Can you work these out from the model? Positions are in its coordinate system, mm. Face numbers are marked on the shaded views. Round coordinates to 2 decimals unless told otherwise and drop trailing zeros. Order: outer loops, then holes, each group sorted by start corner. A loop starts at its lowest first (then second) coordinate and runs counter-clockwise, first axis right, second up. Notation, with made-up numbers: (38.25, 8) -> (53.25, 8) arc R18 ccw to (53.25, 29) -> close; hole circle Ø8 at (11, -3). An arc over 180 degrees is marked (long way). Use a Markdown table: item, result. Add a question column.
Q1. If we section it at B-B on z = -4: List the corners of the cut face in (x, y) for me.
Q2. I need wall thicknesses on line 1 along Y through (x, z) = (0, -7.5); line 2 along Z through (x, y) = (0.05, 0.5); line 3 along Z through (x, y) = (-0.7, -1.6). Which ranges of each line are inside material? Lowest first, please. Write a range as [from, to].
Q3. We'd pull the mould along X, two halves only. Please class the marked faces 1, 2, 3 and 4: +X half, -X half, draft (parallel to the pull), parting line (faces both ways), or undercut.
Q4. If we section it at D-D on z = 7.75: List the corners of the cut face in (x, y) for me.
Q5. If we section it at C-C on y = 0.6: List the corners of the cut face in (x, z) for me.
Q6. If we section it at A-A on x = 0: List the corners of the cut face in (y, z) for me.
Q7. I'm going to push flat-ended pins straight in: pin 1 Ø1.5 at (x, y) = (2, 1.5) entering from +Z; pin 2 Ø0.8 at (x, y) = (0, -0.5) entering from -Z; pin 3 Ø2 at (y, z) = (0.5, -10) entering from +X. Where does each tip first touch, or does it pass through?
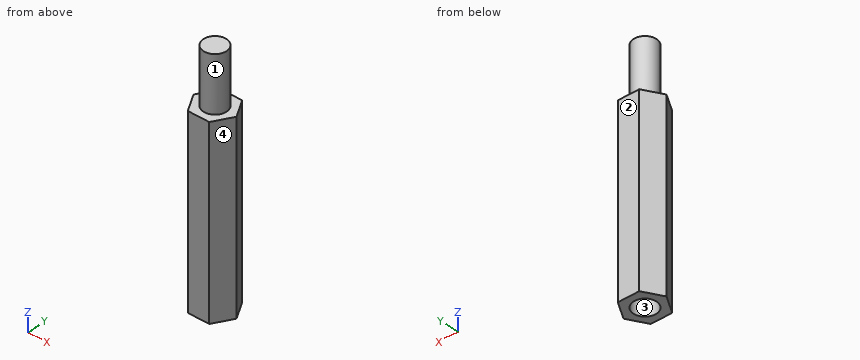
Autodesk Fusion 360 part; units mm, degrees
sketch "Sketch1" plane through (0, 0, 0) normal (0, 0, 1) x (1, 0, 0)
  circle A0 centre (0, 0) radius 1.25
  line L0 (2.3094, 0) -> (1.1547, 2)
  line L1 (1.1547, 2) -> (-1.1547, 2)
  line L2 (-1.1547, 2) -> (-2.3094, 0)
  line L3 (-2.3094, 0) -> (-1.1547, -2)
  line L4 (-1.1547, -2) -> (1.1547, -2)
  line L5 (1.1547, -2) -> (2.3094, 0)
  dimension "d1" = 2.5
  dimension "d21" = 2
extrude "Extrude6" add sketch "Sketch1" along normal blind 6
extrude "Extrude7" add sketch "Sketch1" along normal blind 7 from surface at 5 contours A0
thread "Thread1" thread offset 0 thread length 10
thread "Thread2" thread offset 0 thread length 10
move_face "OffsetFaces2" offset 14 1 faces at (-1.499, 0.9014, 0)
equation "d31 = 1.3 mm + 24 mm - 7.3 mm - 4 mm"
Answer below:
| question | item | result |
|---|---|---|
| 1 | outline | (-2.31, 0) -> (-1.15, -2) -> (1.15, -2) -> (2.31, 0) -> (1.15, 2) -> (-1.15, 2) -> close; hole circle Ø2.5 at (0, 0) |
| 2 | line 1 | [-2, -1.25], [1.25, 2] |
| 2 | line 2 | [5, 12] |
| 2 | line 3 | [-14, 6] |
| 3 | face 1 | parting line |
| 3 | face 2 | draft |
| 3 | face 3 | undercut |
| 3 | face 4 | +X half |
| 4 | outline | circle Ø2.5 at (0, 0) |
| 5 | outline | (-1.96, -14) -> (-1.1, -14) -> (-1.1, 5) -> (1.1, 5) -> (1.1, -14) -> (1.96, -14) -> (1.96, 6) -> (1.1, 6) -> (1.1, 12) -> (-1.1, 12) -> (-1.1, 6) -> (-1.96, 6) -> close |
| 6 | outline | (-2, -14) -> (-1.25, -14) -> (-1.25, 5) -> (1.25, 5) -> (1.25, -14) -> (2, -14) -> (2, 6) -> (1.25, 6) -> (1.25, 12) -> (-1.25, 12) -> (-1.25, 6) -> (-2, 6) -> close |
| 7 | pin 1 | z = 6 |
| 7 | pin 2 | z = 5 |
| 7 | pin 3 | x = 2.31 |
